Input: part model. Units: mm. Frame: model coordinates. Face numbers are marked on the shaded views. Coordinates: 2 decimals unless noted, no trailing zeros. Loops run counter-clockwise (first coordinate to the right, second up) from the corner with the lowest first, then second, coordinate; pieces in that order, holes last. Notation, with made-up numbers: (83, 16) - (105, 16) arc R35 ccw to (105, 48) - close; hole circle Ø7 at (-35, 83). An arc over 180 degrees is marked (long way). Use one line per item in the form item = value.
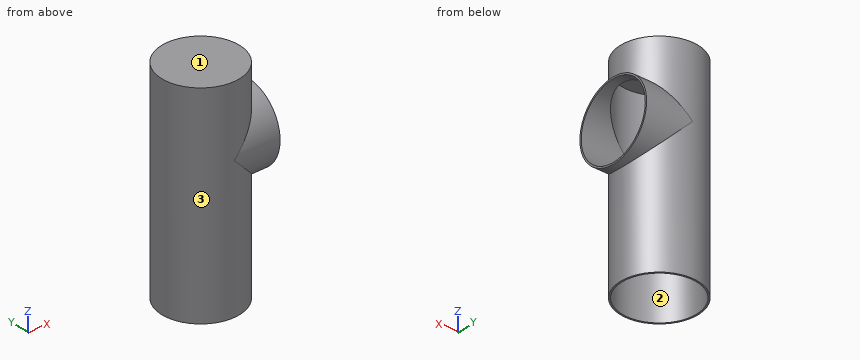
Autodesk Inventor part; units mm, degrees
ref_plane "YZ Plane" through (0, 0, 0) normal (1, 0, 0) x (0, 1, 0)
ref_plane "XZ Plane" through (0, 0, 0) normal (0, 1, 0) x (-1, 0, 0)
ref_plane "XY Plane" through (0, 0, 0) normal (0, 0, 1) x (1, 0, 0)
sketch "Sketch1" plane through (0, 0, 0) normal (0, 0, 1) x (1, 0, 0)
  circle A0 centre (3.175, -9.6512) radius 3.175
  circle A1 centre (3.175, 9.6512) radius 3.175
  circle A2 centre (3.175, -9.6512) radius 3.048
  point P0 (0, 0)
  dimension "d0" = 6.096
extrude "Extrusion1" add sketch "Sketch1" along normal blind 16.51 contours A0
ref_plane "Work Plane1" through (0, 0, 298.4246) normal (1, 0, 0) x (0, 0, 1)
sketch "Sketch2" plane through (0, 0, 298.4246) normal (1, 0, 0) x (0, 0, 1)
  point P0 (-298.4246, 0)
ref_plane "Work Plane2" through (6.985, -9.6512, 9.8182) normal (-1, 0, 0) x (0, 0, 1)
sketch "Sketch3" plane through (6.985, -9.6512, 9.8182) normal (-1, 0, 0) x (0, 0, 1)
  circle A0 centre (1.5875, 0) radius 3.175
  circle A1 centre (1.5875, 0) radius 1.143
  point P0 (-9.8182, 9.6512)
extrude "Extrusion2" cut sketch "Sketch3" along normal blind 3.81 contours A0 | A1
sketch "Sketch4" plane through (3.175, -9.6512, 9.8182) normal (1, 0, 0) x (0, 0, -1)
  arc A0 (-1.5875, 3.175) -> (-1.5875, -3.175) centre (-1.5875, 0) ccw
  circle A1 centre (-1.5875, 0) radius 3.175
  circle A2 centre (-1.5875, 0) radius 3.048
  point P0 (9.8182, 9.6512)
  dimension "d6" = 6.35
  dimension "d7" = 6.096
extrude "Extrusion3" add sketch "Sketch4" along normal blind 3.81
sketch "Sketch5" plane through (3.175, -9.6512, 9.8182) normal (-1, 0, 0) x (0, 0, 1)
  point P0 (-9.8182, 9.6512)
sketch "Sketch6" plane through (3.175, -9.6512, 16.51) normal (0, 0, 1) x (1, 0, 0)
  circle A0 centre (0, 0) radius 3.048
  circle A1 centre (0, 0) radius 3.175
  point P0 (-3.175, 9.6512)
extrude "Extrusion4" cut sketch "Sketch6" against normal through all contours A0
extrude "Extrusion5" add sketch "Sketch6" along normal blind 0.635 contours A0 | A1
properties part number "topwaterpipes"
Q1. Cut plane A-A, the plane y = -10.25. Return loops of the section in (x, z) (3 decimals), then the cut area to 3 significant figures.
Check values:
outline = (0.057, 0) - (0.186, 0) - (0.186, 16.51) - (6.164, 16.51) - (6.164, 14.394) - (6.985, 14.394) - (6.985, 14.524) - (6.293, 14.524) - (6.293, 17.145) - (0.057, 17.145) - close; (6.164, 0) - (6.293, 0) - (6.293, 8.288) - (6.985, 8.288) - (6.985, 8.417) - (6.164, 8.417) - close
area = 7.64 mm²
Q2. Cut plane B-B, the plane x = 5.5. Return loops of the section in (y, z) (3 decimals).
Check values:
outline = (-11.813, 0) - (-11.622, 0) - (-11.622, 9.081) arc R3.048 cw to (-11.622, 13.731) - (-11.622, 16.51) - (-7.68, 16.51) - (-7.68, 13.731) arc R3.048 cw to (-7.68, 9.081) - (-7.68, 0) - (-7.489, 0) - (-7.489, 9.081) arc R3.175 ccw to (-7.489, 13.731) - (-7.489, 17.145) - (-11.813, 17.145) - (-11.813, 13.731) arc R3.175 ccw to (-11.813, 9.081) - close
Q3. Cut plane D-D, the plane z = 4.75. Return loops of the section in (x, y) (3 decimals), then the cut area to 3 significant figures.
Check values:
outline = circle Ø6.35 at (3.175, -9.651); hole circle Ø6.096 at (3.175, -9.651)
area = 2.48 mm²
Q4. Ray query, line 1 along Z through (x, y) = (5.5, -8) (3 decimals); line 2 along Y through (x, z) = (0.5, 1.5); line 3 along Y through (x, z) = (0.75, 4.5). Return the intervals inside material, ascending. Write a range as [from, to].
Check values:
line_1 = [16.51, 17.145]
line_2 = [-11.36, -11.11], [-8.19, -7.94]
line_3 = [-11.7, -11.5], [-7.8, -7.6]
Q5. Cut plane C-C, the plane y = -7.25. Return loops of the section in (x, z) (3 decimals), then the cut area to 3 significant figures.
Check values:
outline = (1.098, 0) - (1.298, 0) - (1.298, 16.51) - (5.052, 16.51) - (5.052, 13.283) - (6.985, 13.283) - (6.985, 13.483) - (5.252, 13.483) - (5.252, 17.145) - (1.098, 17.145) - close; (5.052, 0) - (5.252, 0) - (5.252, 9.328) - (6.985, 9.328) - (6.985, 9.528) - (5.052, 9.528) - close
area = 9.18 mm²
Q6. Pull-direction query (X, two-part tool) for the marked faces 1, 2 and 3; classes: pulls with the +X half, pulls with the -X half, needs draft (parallel to the pull), parting line crosses it, or undercut.
Check values:
face_1 = needs draft
face_2 = undercut
face_3 = parting line crosses it
Q7. First-contact query: P1, Ø3, axis at x = 6, z = 6, coming from the -Y side. Flat tip, straight axial feed; report the tip coordinate or a pass-through.
Check values:
P1 = -12.54
